Autodesk Inventor part; units mm, degrees
ref_plane "Work Plane2" through (405.4179, -139.067, 0) normal (-0.9848, 0.1736, 0) x (0, 0, 1)
ref_plane "YZ Plane" through (0, 0, 0) normal (1, 0, 0) x (0, 1, 0)
ref_plane "XZ Plane" through (0, 0, 0) normal (0, 1, 0) x (-1, 0, 0)
sketch "Sketch1" plane through (0, 0, 0) normal (0, 0, 1) x (1, 0, 0)
  ellipse E0 centre (0, 0) end of major axis (0, 330) minor radius 450 (0, -330) -> (0, 330) ccw
  ellipse E1 centre (0, 0) end of major axis (420, 0) minor radius 300 (0, -300) -> (0, 300) ccw
  line L0 (0, 300) -> (0, 330)
  line L1 (0, -300) -> (0, -330)
  line L2 (420, 0) -> (450, 0)
  dimension "d0" = 420
  dimension "d1" = 450
  dimension "d2" = 300
  dimension "d3" = 330
extrude "Extrusion1" add sketch "Sketch1" along normal blind 160
sketch "Sketch3" plane through (0, 0, 0) normal (0, 0, -1) x (-1, 0, 0)
  ellipse E0 centre (0, 0) end of major axis (420, 0) minor radius 300 (0, 300) -> (0, -300) ccw
  line L0 (-410.6033, 63.104) -> (-375.8737, -133.8576)
  line L1 (-375.8737, -133.8576) -> (-428.5073, -143.1383)
  line L2 (-428.5073, -143.1383) -> (-456.291, 14.4309)
  line L3 (0, 300) -> (0, -300)
  ellipse E1 centre (0, 0) end of major axis (450, 0) minor radius 330 (0, 330) -> (0, -330) ccw
  line L4 (-456.291, 14.4309) -> (-439.6592, 70.3382)
  line L5 (-428.5073, -143.1383) -> (-336.4493, -219.1451)
  line L6 (-336.4493, -219.1451) -> (-375.8737, -133.8576)
  line L7 (-410.6033, 63.104) -> (-439.6592, 70.3382)
  line L8 (-393.2385, -35.3768) -> (260.9914, 90.2506)
  line L9 (260.9914, 90.2506) -> (260.9914, 44.7879)
  line L10 (260.9914, 44.7879) -> (0, 40.1342)
  dimension "d8" = 200
  dimension "d9" = 10
  dimension "d12" = 45.4627
  dimension "d13" = 160
extrude "Extrusion2" add sketch "Sketch3" against normal blind 160 contours L0 E0
sketch "Sketch7" plane through (0, 0, 160) normal (0, 0, 1) x (1, 0, 0)
  ellipse E0 centre (0, 0) end of major axis (-450, 0) minor radius 330 (0, -330) -> (0, 330) ccw
  line L0 (0, 330) -> (0, 300)
  ellipse E1 centre (0, 0) end of major axis (-420, 0) minor radius 300 (410.6033, 63.104) -> (0, 300) ccw
  line L1 (410.6033, 63.104) -> (375.8737, -133.8576)
  ellipse E2 centre (0, 0) end of major axis (-420, 0) minor radius 300 (0, -300) -> (375.8737, -133.8576) ccw
  line L2 (0, -300) -> (0, -330)
  line L3 (0, -300) -> (0, 300)
extrude "Extrusion6" add sketch "Sketch7" along normal blind 5
ref_plane "Work Plane2" through (405.4179, -139.067, 0) normal (-0.9848, 0.1736, 0) x (0, 0, 1)
sketch "Sketch8" plane through (405.4179, -139.067, 0) normal (-0.9848, 0.1736, 0) x (0, 0, 1)
  circle A0 centre (80.8275, 83.1092) radius 366.3368
  point P0 (0, 66.5542)
extrude "Extrusion7" cut sketch "Sketch8" against normal blind 200
sketch "Sketch9" plane through (0, 300, 0) normal (-1, 0, 0) x (0, 0, 1)
  line L0 (0, -630) -> (0, -444.7158)
  line L1 (0, -630) -> (215, -630)
  line L2 (215, -630) -> (215, -680)
  line L3 (215, -680) -> (0, -680)
  line L4 (0, -680) -> (0, -630)
  line L5 (165, -235.481) -> (165, 30)
  line L6 (215, -630) -> (165, -630)
  line L7 (165, -630) -> (165, 30)
  line L8 (165, 30) -> (215, 30)
  line L9 (215, 30) -> (215, -630)
  line L10 (215, 30) -> (0, 30)
  line L11 (0, 30) -> (0, 80)
  line L12 (0, 80) -> (215, 80)
  line L13 (215, 80) -> (215, 30)
  circle A0 centre (190, -655) radius 4.5
  circle A1 centre (140, -655) radius 4.5
  circle A2 centre (90, -655) radius 4.5
  circle A3 centre (40, -655) radius 4.5
  circle A4 centre (190, -605) radius 4.5
  circle A5 centre (190, -555) radius 4.5
  circle A6 centre (190, -505) radius 4.5
  circle A7 centre (190, -455) radius 4.5
  circle A8 centre (190, -405) radius 4.5
  circle A9 centre (190, -355) radius 4.5
  line L14 (215, -300) -> (251.9501, -300)
  circle A10 centre (190, 55) radius 4.5
  circle A11 centre (140, 55) radius 4.5
  circle A12 centre (90, 55) radius 4.5
  circle A13 centre (40, 55) radius 4.5
  circle A14 centre (190, 5) radius 4.5
  circle A15 centre (190, -45) radius 4.5
  circle A16 centre (190, -95) radius 4.5
  circle A17 centre (190, -145) radius 4.5
  circle A18 centre (190, -195) radius 4.5
  circle A19 centre (190, -245) radius 4.5
  point P0 (0, -300)
  dimension "d34" = 50
  dimension "d35" = 50
  dimension "d36" = 50
  dimension "d39" = 9
  dimension "d40" = 25
  dimension "d41" = 25
  dimension "d44" = 50
  dimension "d51" = 50
sketch "Sketch10" plane through (0, 300, 0) normal (-1, 0, 0) x (0, 0, 1)
  point P0 (0, -300)
extrude "Extrusion8" add sketch "Sketch9" against normal blind 5
sketch "Sketch11" plane through (405.4179, -139.067, 0) normal (0.9848, -0.1736, 0) x (0, 0, -1)
  circle A0 centre (-70, 74.2641) radius 35
  circle A1 centre (-70, 129.2641) radius 4.5
  line L0 (0, -5.7359) -> (-165, -5.7359)
  line L1 (-165, 206.7266) -> (0, 206.7266)
  line L2 (-165, -5.7359) -> (-165, 206.7266)
  circle A2 centre (-108.8909, 113.155) radius 4.5
  circle A3 centre (-125, 74.2641) radius 4.5
  circle A4 centre (-108.8909, 35.3732) radius 4.5
  circle A5 centre (-70, 19.2641) radius 4.5
  circle A6 centre (-31.1091, 35.3732) radius 4.5
  circle A7 centre (-15, 74.2641) radius 4.5
  circle A8 centre (-31.1091, 113.155) radius 4.5
  line L3 (0, 206.7266) -> (0, -5.7359)
  point P0 (0, 66.5542)
  dimension "d56" = 70
  dimension "d57" = 9
  dimension "d58" = 55
  dimension "d59" = 212.4625
  dimension "d64" = 360
  dimension "d66" = 0
  dimension "d69" = 80
  dimension "d70" = 70
extrude "Extrusion9" cut sketch "Sketch11" against normal blind 50 contours A0 | A1 | A2 | A3 | A4 | A5 | A6 | A7 | A8
properties part number "eggshellCorePrinted" material "GFRC"
Can you work these out from the model? Positions are in its coordinate system, mm. A direction names the side the tool comes from. Coordinates: 2 decimals unless noted, no trailing zeros. Return JSON: item names as keys, results as strings. Group by question number.
Item 1: We'd pull the mould along X, two halves only. Please class faces 3 (the face through (393.48, -34, 96.66)), 4 (the face through (393.9, -119.22, 65.84)), 5 (the face through (5, 5, 178)), 6 (the face through (172, 5, 165)): pulls with the +X half, pulls with the -X half, needs draft (parallel to the pull), parting line crosses it, or undercut.
Item 2: Which directions (+Z, -Z, +X, -X, +Y, -Y) give clear straight access to the entire face, cutting with the end or side of a thin tool? Please do faces 1 (the face through (157, 4, 160)), 2 (the face through (403.448, -65.06, 10.843)).
Item 3: I'm going to push flat-ended pins straight in: pin 1 Ø5.5 at (y, z) = (-355, 40) entering from -X; pin 2 Ø4 at (x, y) = (133, 197) entering from +Z; pin 3 Ø14.5 at (y, z) = (-355, 190) entering from +X; pin 4 Ø10 at (x, z) = (341.5, 113) entering from -Y. Where does each tip first touch, or does it pass through?
Item 4: Please list where these lines run through material, in increasing order: probe 1 along Z at (x, y) = (2.65, -305); probe 2 along Z at (x, y) = (419, 48.5); probe 3 along Y at (x, z) = (213, 87).
Return value:
{
 "1": {"face 3": "pulls with the -X half", "face 4": "undercut", "face 5": "pulls with the +X half", "face 6": "needs draft"},
 "2": {"face 1": "-Z, -X", "face 2": "none"},
 "3": {"pin 1": "passes through", "pin 2": "stops at z = 165", "pin 3": "stops at x = 5", "pin 4": "stops at y = -219.1"},
 "4": {"probe 1": "z = 0 to 185.5, 194.5 to 215", "probe 2": "z = 0 to 165", "probe 3": "y = -290.69 to -258.56, 258.56 to 290.69"}
}
